Geometry check sheet. Reference: the model listing, model coordinates, mm. A direction names the side the tool comes from. Round coordinates to 2 decimals unless told otherwise and drop trailing zeros. Loops run counter-clockwise (first coordinate to the right, second up) from the corner with the lowest first, then second, coordinate; pieces in that order, holes last. Notation, with made-up numbers: M -21,73 L 13,73 A23 cw 13,82 Z; hole C -13,-38.75 d11. An arc over 180 degrees is marked long. Write item = value, one per line.
from build123d import *

# Parameters (mm, degrees)
SKETCH_1_R      = 14.5
EXTRUDE_1_DEPTH = 42.6
SKETCH_3_W      = 1.5
SKETCH_3_H      = 17.5


with BuildPart() as part:
    # 草圖1 → 填料-伸長1 (new body)
    with BuildSketch(Plane.XY):
        Circle(SKETCH_1_R)
    extrude(amount=EXTRUDE_1_DEPTH)

    # 草圖3 → 除料-旋轉1 (revolve, cut)
    with BuildSketch(Plane(origin=(0, 0, 0), x_dir=(1, 0, 0), z_dir=(0, 1, 0))):
        Polygon((-4.5, 0), (-13, -6.6), (-13, -18.3), (-14.5, -18.3), (-14.5, 0), align=None)
        with Locations((-13.75, -33.85)):
            Rectangle(SKETCH_3_W, SKETCH_3_H)
    revolve(axis=Axis((0, 0, 0), (0, 0, 1)), mode=Mode.SUBTRACT)


solid = part.part
(1) Material ranges on line 1 along Z through (x, y) = (3, -13.5); line 2 along Y through (x, z) = (-6.5, 10.5); line 3 along Z through (x, y) = (4.5, 8.25), recorded low to high. Write a range as from..to.
Result set:
line_1 = 18.3..25.1
line_2 = -11.26..11.26
line_3 = 3.8..42.6
(2) Depth check by flat-ended pin: pin 1 Ø3 at (x, z) = (-10.5, 13) entering from +Y; pin 2 Ø12 at (y, z) = (-7.5, 15.5) entering from -X; pin 3 Ø1 at (x, z) = (-8.5, 15.5) entering from -Y. Enter the tip coordinate at first touch or a pass-through.
Result set:
pin_1 = 9.38
pin_2 = -14.33
pin_3 = -10.25
(3) Sectioned sample at D-D on z = 22.5. Record the cut outline in (x, y).
Result set:
outline = C 0,0 d29
(4) Sectioned sample at A-A on x = 0. Record the cut outline in (y, z), then the cut area to 3 significant figures.
Result set:
outline = M -14.5,18.3 L -13,18.3 L -13,6.6 L -4.5,0 L 4.5,0 L 13,6.6 L 13,18.3 L 14.5,18.3 L 14.5,25.1 L 13,25.1 L 13,42.6 L -13,42.6 L -13,25.1 L -14.5,25.1 Z
area = 1,070 mm2
(5) Tool access check on faces 1 (the cylindrical face through (10.316, 7.91, 33.728)), 2 (the cylindrical face through (6.691, -12.864, 21.652)), 3 (the cylindrical face through (10.316, 7.91, 12.532)). Record the directions out of +Z, -Z, +X, -X, +Y, -Y that give a thin tool (end or side, any length) a straight path to the whole face; none if there is none.
Result set:
face_1 = +Z
face_2 = +Z, -Z
face_3 = -Z
(6) Sectioned sample at C-C on z = 30. Record the cut outline in (x, y).
Result set:
outline = C 0,0 d26
